Can you work these out from the model? Positions are in its coordinate system, mm. A direction names the side the tool comes from. Give positions to 0.01 mm unless a question says otherwise; leave off trailing zeros. Loops run counter-clockwise (first coordinate to the right, second up) from the corner with the lowest first, then second, coordinate; pieces in that order, holes last.
from build123d import *

# Parameters (mm, degrees)
BOSS_EXTRUDE7_DEPTH                          = 17
BOSS_EXTRUDE7_DEPTH_BACK                     = 17
SKETCH1_R                                    = 1.45
SKETCH34_W                                   = 28.4
SKETCH34_H                                   = 7.5
CUT_EXTRUDE11_DEPTH                          = 37.521397837
SKETCH35_R                                   = 5
CUT_EXTRUDE12_DEPTH                          = 25.542055741
CSK_FOR_M3_HEX_SOCKET_COUNTERSUNK_CA_2_COUNT = 2
CSK_FOR_M3_HEX_SOCKET_COUNTERSUNK_CA_2_PITCH = 16.5
CSK_FOR_M3_HEX_SOCKET_COUNTERSUNK_CA_3_COUNT = 2
CSK_FOR_M3_HEX_SOCKET_COUNTERSUNK_CA_3_PITCH = 18
CSK_FOR_M3_HEX_SOCKET_COUNTERSUNK_CA_4_COUNT = 2
CSK_FOR_M3_HEX_SOCKET_COUNTERSUNK_CA_4_PITCH = 24.418230894
FILLET5_R                                    = 1
SKETCH41_W                                   = 28.5
SKETCH41_H                                   = 0.4
CUT_EXTRUDE13_DEPTH                          = 40.895175147
BOSS_EXTRUDE8_START                          = 5
BOSS_EXTRUDE8_DEPTH                          = 5
SKETCH48_R                                   = 1.4
CUT_EXTRUDE14_DEPTH                          = 5
SKETCH49_R                                   = 2.55
CUT_EXTRUDE15_DEPTH                          = 2


with BuildPart() as part:
    # Sketch1 → Boss-Extrude7 (new, two sides: drawn at the far end of the back side and taken through both)
    # profile 1 of 3: a face of its own
    with BuildSketch(Plane.XY.offset(-BOSS_EXTRUDE7_DEPTH_BACK)):
        Polygon((-14.25, 15.25), (-14.25, 11.25), (-8.25, 11.25), (-8.25, 12.25), (8.25, 12.25), (8.25, 11.25), (14.25, 11.25), (14.25, 15.25), align=None)
    # profile 2 of 3: a face of its own
    with BuildSketch(Plane.XY.offset(-BOSS_EXTRUDE7_DEPTH_BACK)):
        with BuildLine():
            Line((14.25, 4.75), (14.25, 11.25))
            Line((14.25, 11.25), (8.25, 11.25))
            Line((8.25, 11.25), (8.25, 8.011710179))
            ThreePointArc((8.25, 8.011710179), (9.502581542, 6.476954843), (10.473180033, 4.75))
            Line((10.473180033, 4.75), (14.25, 4.75))
        make_face()
        with Locations((11, 8)):
            Circle(SKETCH1_R, mode=Mode.SUBTRACT)
    # profile 3 of 3: a face of its own
    with BuildSketch(Plane.XY.offset(-BOSS_EXTRUDE7_DEPTH_BACK)):
        with BuildLine():
            Line((-8.25, 11.25), (-14.25, 11.25))
            Line((-14.25, 11.25), (-14.25, 4.75))
            Line((-14.25, 4.75), (-10.473180033, 4.75))
            ThreePointArc((-10.473180033, 4.75), (-9.502581542, 6.476954843), (-8.25, 8.011710179))
            Line((-8.25, 8.011710179), (-8.25, 11.25))
        make_face()
        with Locations((-11, 8)):
            Circle(SKETCH1_R, mode=Mode.SUBTRACT)
    extrude(amount=BOSS_EXTRUDE7_DEPTH + BOSS_EXTRUDE7_DEPTH_BACK)

    # Sketch34 → Cut-Extrude11 (cut, through all)
    with BuildSketch(Plane.ZY.offset(14.25)):
        with Locations((0, 8.5)):
            Rectangle(SKETCH34_W, SKETCH34_H)
    extrude(amount=-CUT_EXTRUDE11_DEPTH, mode=Mode.SUBTRACT)

    # Sketch35 → Cut-Extrude12 (cut, through all)
    with BuildSketch(Plane(origin=(0, 15.25, 0), x_dir=(1, 0, 0), z_dir=(0, 1, 0))):
        with Locations(Location((0, 0, 0), (0, 0, 270))):
            Circle(SKETCH35_R)
    extrude(amount=-CUT_EXTRUDE12_DEPTH, mode=Mode.SUBTRACT)

    # Sketch40 → CSK for M3 Hex Socket Countersunk Cap Sc (revolve, cut)
    with BuildSketch(Plane(origin=(-8.25, 12.25, 9), x_dir=(0, 0, -1), z_dir=(1, 0, 0))):
        Polygon((0, 0), (0, 3), (1.7, 3), (1.7, 1.66), (3.36, 0), align=None)
    csk_for_m3_hex_socket_countersunk_cap_sc = revolve(axis=Axis((-8.25, 5.9, 9), (0, 1, 0)), mode=Mode.SUBTRACT)

    # CSK for M3 Hex Socket Countersunk Ca 2: CSK for M3 Hex Socket Countersunk Cap Sc ×2
    with Locations(*[(i * CSK_FOR_M3_HEX_SOCKET_COUNTERSUNK_CA_2_PITCH, 0, 0) for i in range(1, CSK_FOR_M3_HEX_SOCKET_COUNTERSUNK_CA_2_COUNT)]):
        add(csk_for_m3_hex_socket_countersunk_cap_sc, mode=Mode.SUBTRACT)

    # CSK for M3 Hex Socket Countersunk Ca 3: CSK for M3 Hex Socket Countersunk Cap Sc ×2
    with Locations(*[(0, 0, -i * CSK_FOR_M3_HEX_SOCKET_COUNTERSUNK_CA_3_PITCH) for i in range(1, CSK_FOR_M3_HEX_SOCKET_COUNTERSUNK_CA_3_COUNT)]):
        add(csk_for_m3_hex_socket_countersunk_cap_sc, mode=Mode.SUBTRACT)

    # CSK for M3 Hex Socket Countersunk Ca 4: CSK for M3 Hex Socket Countersunk Cap Sc ×2
    with Locations(*[Vector(0.6757246285173466, 0, -0.7371541402007413) * (i * CSK_FOR_M3_HEX_SOCKET_COUNTERSUNK_CA_4_PITCH) for i in range(1, CSK_FOR_M3_HEX_SOCKET_COUNTERSUNK_CA_4_COUNT)]):
        add(csk_for_m3_hex_socket_countersunk_cap_sc, mode=Mode.SUBTRACT)

    # Fillet5
    fillet5_edges = [part.edges().sort_by_distance(p)[0] for p in [
        (14.25, 15.25, 0),
        (0, 15.25, -17),
        (0, 15.25, 17),
    ]]
    fillet(fillet5_edges, radius=FILLET5_R)

    # Sketch41 → Cut-Extrude13 (cut, through all)
    with BuildSketch(Plane.XY.offset(17)):
        with Locations((0, 4.95)):
            Rectangle(SKETCH41_W, SKETCH41_H)
    extrude(amount=-CUT_EXTRUDE13_DEPTH, mode=Mode.SUBTRACT)

    # Sketch46 → Boss-Extrude8 (add)
    with BuildSketch(Plane.ZY.offset(14.25).offset(BOSS_EXTRUDE8_START)):
        Polygon((17, -22.75), (17, 5.15), (14.2, 5.15), (14.2, 12.25), (-14.2, 12.25), (-14.2, 5.15), (-17, 5.15), (-17, -22.75), align=None)
        with BuildLine():
            ThreePointArc((-16, 15.25), (-16.707106781, 14.957106781), (-17, 14.25))
            Line((-17, 14.25), (-17, 5.15))
            Line((-17, 5.15), (-14.2, 5.15))
            Line((-14.2, 5.15), (-14.2, 12.25))
            Line((-14.2, 12.25), (14.2, 12.25))
            Line((14.2, 12.25), (14.2, 5.15))
            Line((14.2, 5.15), (17, 5.15))
            Line((17, 5.15), (17, 14.25))
            ThreePointArc((17, 14.25), (16.707106781, 14.957106781), (16, 15.25))
            Line((16, 15.25), (-16, 15.25))
        make_face()
    extrude(amount=-BOSS_EXTRUDE8_DEPTH)

    # Sketch48 → Cut-Extrude14 (cut)
    with BuildSketch(Plane.ZY.offset(19.25)):
        with Locations(Location((-10, -11.75, 0), (0, 0, 270))):
            Circle(SKETCH48_R)
        with Locations(Location((10, -11.75, 0), (0, 0, 270))):
            Circle(SKETCH48_R)
        with Locations(Location((10, 4.25, 0), (0, 0, 270))):
            Circle(SKETCH48_R)
        with Locations(Location((-10, 4.25, 0), (0, 0, 270))):
            Circle(SKETCH48_R)
    extrude(amount=-CUT_EXTRUDE14_DEPTH, mode=Mode.SUBTRACT)

    # Sketch49 → Cut-Extrude15 (cut)
    with BuildSketch(Plane(origin=(-14.25, 0, 0), x_dir=(0, 0, -1), z_dir=(1, 0, 0))):
        with Locations(Location((-10, -11.75, 0), (0, 0, 90))):
            Circle(SKETCH49_R)
        with Locations(Location((10, -11.75, 0), (0, 0, 90))):
            Circle(SKETCH49_R)
        with Locations(Location((10, 4.25, 0), (0, 0, 90))):
            Circle(SKETCH49_R)
        with Locations(Location((-10, 4.25, 0), (0, 0, 90))):
            Circle(SKETCH49_R)
    extrude(amount=-CUT_EXTRUDE15_DEPTH, mode=Mode.SUBTRACT)


solid = part.part
(1) Suppose I cut it at A-A on z = 0. List the corners of the cut face in (x, y) for me, plus the area to 3 significant figures.
Returned:
outline: (-19.25, -22.75) - (-14.25, -22.75) - (-14.25, 12.25) - (-5, 12.25) - (-5, 15.25) - (-19.25, 15.25) - close; (5, 12.25) - (14.25, 12.25) - (14.25, 14.25) arc R1 ccw to (13.25, 15.25) - (5, 15.25) - close
area: 245 mm2
(2) Which directions (+Z, -Z, +X, -X, +Y, -Y) give clear straight access to the entire face, cutting with the end or side of a thin tool? Please do faces 4 (the cylindrical face through (-9.39, 6.64, -15.62)), 5 (the cylindrical face through (-15.24, -12.3, 7.51)), 6 (the flat face through (12, 5.15, -16)).
Returned:
face 4: +Z, -Z, -Y
face 5: +X
face 6: +Z, -Z, +X, -Y
(3) Suppose I cut it at C-C on y = 4.25. List the corners of the cut face in (x, z) for me.
Returned:
outline: (-19.25, -17) - (-14.25, -17) - (-14.25, -12.55) - (-16.25, -12.55) - (-16.25, -11.4) - (-19.25, -11.4) - close; (-19.25, -8.6) - (-16.25, -8.6) - (-16.25, -7.45) - (-14.25, -7.45) - (-14.25, 7.45) - (-16.25, 7.45) - (-16.25, 8.6) - (-19.25, 8.6) - close; (-19.25, 11.4) - (-16.25, 11.4) - (-16.25, 12.55) - (-14.25, 12.55) - (-14.25, 17) - (-19.25, 17) - close
(4) Suppose I cut it at B-B on x = -4. List the corners of the cut face in (y, z) for me, plus the area to 3 significant figures.
Returned:
outline: (12.25, -17) - (14.25, -17) arc R1 ccw to (15.25, -16) - (15.25, -3) - (12.25, -3) - close; (12.25, 3) - (15.25, 3) - (15.25, 16) arc R1 ccw to (14.25, 17) - (12.25, 17) - close
area: 83.6 mm2
(5) Suppose I cut it at D-D on x = -13. List the corners of the cut face in (y, z) for me.
Returned:
outline: (5.15, -17) - (14.25, -17) arc R1 ccw to (15.25, -16) - (15.25, 16) arc R1 ccw to (14.25, 17) - (5.15, 17) - (5.15, 14.2) - (12.25, 14.2) - (12.25, -14.2) - (5.15, -14.2) - close
(6) Will these pins go through, and if not, where does the flat tip stop? P1, Ø1.4, axis at x = -11.5, z = -15, coming from the -Y side; P2, Ø1, axis at x = -13, z = 5.5, coming from the -Y side; P3, Ø2.5, axis at y = 4, z = -9.5, coming from the +X side.
Returned:
P1: stops at y = 5.15
P2: stops at y = 12.25
P3: stops at x = -16.25
(7) Thinking about a two-plate mould opening in X: for faces 1 (the flat face through (-14.25, -5, 0)), 2 (the cylindrical face through (9.91, 14.57, 9.37)), 3 (the flat face through (-12, 5.15, -16)), which applies, pulls with the +X half, pulls with the -X half, needs draft (parallel to the pull), parting line crosses it, or undercut?
Returned:
face 1: pulls with the +X half
face 2: undercut
face 3: needs draft
(8) Please list where these lines run through material, in increasing order: probe 1 along X at (y, z) = (14, -9); probe 2 along Z at (x, y) = (-17.1, 4.25); probe 3 along Y at (x, z) = (-11, -15.5).
Returned:
probe 1: x = -19.25 to -9.95, -6.55 to 6.55, 9.95 to 14.25
probe 2: z = -17 to -11.4, -8.6 to 8.6, 11.4 to 17
probe 3: y = 5.15 to 6.55, 9.45 to 15.25
